Geometry check sheet. Reference: the model listing, model coordinates, mm. Face numbers are marked on the shaded views. Coordinates: 2 decimals unless noted, no trailing zeros. Order: outer loops, then holes, each group sorted by start corner. A loop starts at its lowest first (then second) coordinate and runs counter-clockwise, first axis right, second up. Notation, with made-up numbers: M 16.25,16 L 35.25,16 A21 ccw 35.25,48 Z; hole C 54.25,8.25 d7. An arc over 180 degrees is marked long. One line per item, written item: value. Start each with the question number.
1) Go/stop test with flat-tipped pins: P1, Ø1.8, axis at x = -0.5, y = -1, coming from the -Z side; P2, Ø1, axis at x = 5, z = -3.5, coming from the +Y side. Record where each tip stops, or that it passes through.
2) Draft check along Y on the marked faces 1, 2 and 3. Enter one of: pulls with the +Y half, pulls with the -Y half, needs draft (parallel to the pull), parting line crosses it, or undercut.
3) Thickness scan on L1, parallel to Y at x = 0, z = -3.7; L2, parallel to Y at x = 0, z = -1.85; L3, parallel to X at y = 0.5, z = -1.75. Record the ranges inside material, lowest first. Write a range as from..to.
4) Sectioned sample at C-C, the plane z = -5.5. Enter the section's corners in (x, y), then the cut area to 3 significant figures.
5) Sectioned sample at A-A, the plane y = 0. Enter the section's corners in (x, z).
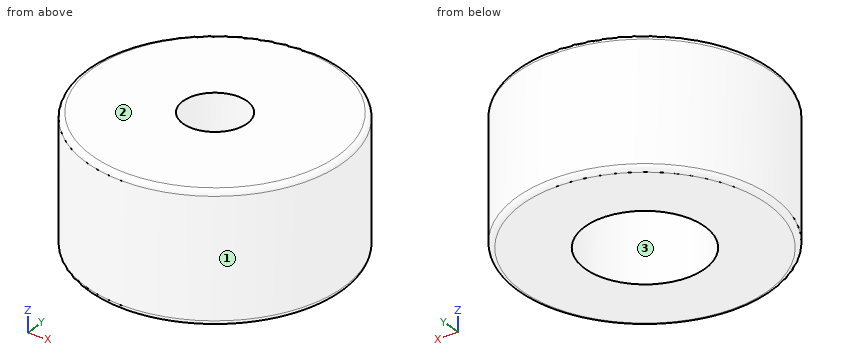
```python
from build123d import *

# Parameters (mm, degrees)
FILLET1_R = 0.254


with BuildPart() as part:
    # Sketch1 → Revolve1 (revolve)
    with BuildSketch(Plane(origin=(0, 0, 0), x_dir=(1, 0, 0), z_dir=(0, 1, 0))):
        Polygon((-1.5875, 0), (-6.35, 0), (-6.35, 6.35), (-2.9718, 6.35), (-2.9718, 2.38125), (-1.5875, 2.38125), align=None)
    revolve(axis=Axis((0, 0, 0), (0, 0, -1)))

    # Fillet1
    fillet1_edges = [part.edges().sort_by_distance(p)[0] for p in [
        (6.35, 0, 0),
        (6.35, 0, -6.35),
    ]]
    fillet(fillet1_edges, radius=FILLET1_R)


solid = part.part
```
Final values:
1. P1: stops at z = -2.38
1. P2: stops at y = 4.48
2. face 1: parting line crosses it
2. face 2: needs draft
2. face 3: undercut
3. L1: y = -6.35..-2.97, 2.97..6.35
3. L2: y = -6.35..-1.59, 1.59..6.35
3. L3: x = -6.33..-1.51, 1.51..6.33
4. outline: C 0,0 d12.7; hole C 0,0 d5.94
4. area: 98.9 mm^2
5. outline: M -6.35,-6.1 A0.25 ccw -6.1,-6.35 L -2.97,-6.35 L -2.97,-2.38 L -1.59,-2.38 L -1.59,0 L -6.1,0 A0.25 ccw -6.35,-0.25 Z; M 1.59,-2.38 L 2.97,-2.38 L 2.97,-6.35 L 6.1,-6.35 A0.25 ccw 6.35,-6.1 L 6.35,-0.25 A0.25 ccw 6.1,0 L 1.59,0 Z
